The model under review builds one solid part; all positions refer to its coordinate system, in mm. Face numbers are marked on the shaded views. A direction names the side the tool comes from. Round coordinates to 2 decimals unless told otherwise and drop trailing zeros. Order: outer loops, then holes, each group sorted by start corner. A loop starts at its lowest first (then second) coordinate and runs counter-clockwise, first axis right, second up. Notation, with made-up numbers: (88, 3.5) -> (120, 3.5) arc R32 ccw to (120, 38.5) -> close; hole circle Ø1 at (-14.75, -12.5). An arc over 180 degrees is marked (long way). Return JSON: item names as keys, results as strings. Group by question number.
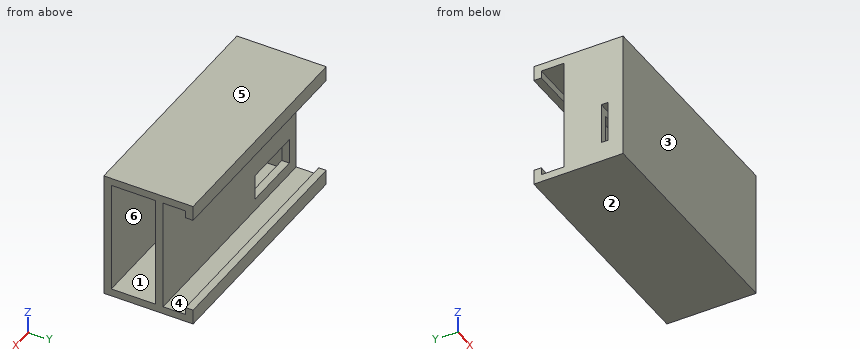
from build123d import *

# Parameters (mm, degrees)
SKETCH1_W            = 155
SKETCH1_H            = 85
BOSS_EXTRUDE1_DEPTH  = 5
SKETCH2_W            = 54
SKETCH2_H            = 35.4
BOSS_EXTRUDE19_DEPTH = 5
SKETCH14_W           = 5
SKETCH14_H           = 35.4
BOSS_EXTRUDE23_DEPTH = 9
SKETCH17_W           = 49
SKETCH17_H           = 4
BOSS_EXTRUDE24_DEPTH = 9
SKETCH18_W           = 49
SKETCH18_H           = 4.5
BOSS_EXTRUDE25_DEPTH = 5
SKETCH19_W           = 17.4
SKETCH19_H           = 4.5
BOSS_EXTRUDE26_DEPTH = 5
SKETCH20_W           = 49
SKETCH20_H           = 4
BOSS_EXTRUDE27_DEPTH = 9
SKETCH21_W           = 49
SKETCH21_H           = 4.5
BOSS_EXTRUDE28_DEPTH = 9
SKETCH24_W           = 40
SKETCH24_H           = 5.3
CUT_EXTRUDE3_DEPTH   = 9
SKETCH26_W           = 155
SKETCH26_H           = 5
BOSS_EXTRUDE29_DEPTH = 54.5
SKETCH27_W           = 155
SKETCH27_H           = 5
BOSS_EXTRUDE30_DEPTH = 75
SKETCH28_W           = 155
SKETCH28_H           = 5
BOSS_EXTRUDE31_DEPTH = 54.5
SKETCH29_W           = 75
SKETCH29_H           = 34.5
BOSS_EXTRUDE32_DEPTH = 5
SKETCH30_W           = 40
SKETCH30_H           = 17
CUT_EXTRUDE4_DEPTH   = 5
SKETCH31_W           = 27.4
SKETCH31_H           = 4.5
CUT_EXTRUDE6_DEPTH   = 5
SKETCH32_W           = 155
SKETCH32_H           = 5
BOSS_EXTRUDE33_DEPTH = 10
SKETCH33_W           = 155
SKETCH33_H           = 5
BOSS_EXTRUDE34_DEPTH = 10


with BuildPart() as part:
    # Sketch1 → Boss-Extrude1 (new body)
    with BuildSketch(Plane(origin=(0, 0, 0), x_dir=(1, 0, 0), z_dir=(0, 1, 0))):
        with Locations((48.537611559, -27.765767023)):
            Rectangle(SKETCH1_W, SKETCH1_H)
    extrude(amount=BOSS_EXTRUDE1_DEPTH)

    # Sketch2 → Boss-Extrude19 (add)
    with BuildSketch(Plane(origin=(0, 5, 0), x_dir=(1, 0, 0), z_dir=(0, 1, 0))):
        with Locations((3.037611559, -12.265767023)):
            Rectangle(SKETCH2_W, SKETCH2_H)
    extrude(amount=BOSS_EXTRUDE19_DEPTH)

    # Sketch14 → Boss-Extrude23 (add)
    with BuildSketch(Plane(origin=(0, 10, 0), x_dir=(1, 0, 0), z_dir=(0, 1, 0))):
        with Locations((27.537611559, -12.265767023)):
            Rectangle(SKETCH14_W, SKETCH14_H)
    extrude(amount=BOSS_EXTRUDE23_DEPTH)

    # Sketch17 → Boss-Extrude24 (add)
    with BuildSketch(Plane(origin=(0, 10, 0), x_dir=(1, 0, 0), z_dir=(0, 1, 0))):
        with Locations((0.537611559, 3.434232977)):
            Rectangle(SKETCH17_W, SKETCH17_H)
    extrude(amount=BOSS_EXTRUDE24_DEPTH)

    # Sketch18 → Boss-Extrude25 (add)
    with BuildSketch(Plane.XY.offset(-1.434232977)):
        with Locations((0.537611559, 16.75)):
            Rectangle(SKETCH18_W, SKETCH18_H)
    extrude(amount=BOSS_EXTRUDE25_DEPTH)

    # Sketch19 → Boss-Extrude26 (add)
    with BuildSketch(Plane.ZY.offset(-25.037611559)):
        with Locations((12.265767023, 16.75)):
            Rectangle(SKETCH19_W, SKETCH19_H)
    extrude(amount=BOSS_EXTRUDE26_DEPTH)

    # Sketch20 → Boss-Extrude27 (add)
    with BuildSketch(Plane(origin=(0, 10, 0), x_dir=(1, 0, 0), z_dir=(0, 1, 0))):
        with Locations((0.537611559, -27.965767023)):
            Rectangle(SKETCH20_W, SKETCH20_H)
    extrude(amount=BOSS_EXTRUDE27_DEPTH)

    # Sketch21 → Boss-Extrude28 (add)
    with BuildSketch(Plane.XY.offset(29.965767023)):
        with Locations((0.537611559, 16.75)):
            Rectangle(SKETCH21_W, SKETCH21_H)
    extrude(amount=-BOSS_EXTRUDE28_DEPTH)

    # Sketch24 → Cut-Extrude3 (cut)
    with BuildSketch(Plane(origin=(0, 19, 0), x_dir=(1, 0, 0), z_dir=(0, 1, 0))):
        with Locations((-0.962388441, -0.915767023)):
            Rectangle(SKETCH24_W, SKETCH24_H)
    extrude(amount=-CUT_EXTRUDE3_DEPTH, mode=Mode.SUBTRACT)

    # Sketch26 → Boss-Extrude29 (add)
    with BuildSketch(Plane(origin=(0, 5, 0), x_dir=(1, 0, 0), z_dir=(0, 1, 0))):
        with Locations((48.537611559, 12.234232977)):
            Rectangle(SKETCH26_W, SKETCH26_H)
    extrude(amount=BOSS_EXTRUDE29_DEPTH)

    # Sketch27 → Boss-Extrude30 (add)
    with BuildSketch(Plane.XY.offset(-9.734232977)):
        with Locations((48.537611559, 37)):
            Rectangle(SKETCH27_W, SKETCH27_H)
    extrude(amount=BOSS_EXTRUDE30_DEPTH)

    # Sketch28 → Boss-Extrude31 (add)
    with BuildSketch(Plane(origin=(0, 5, 0), x_dir=(1, 0, 0), z_dir=(0, 1, 0))):
        with Locations((48.537611559, -67.765767023)):
            Rectangle(SKETCH28_W, SKETCH28_H)
    extrude(amount=BOSS_EXTRUDE31_DEPTH)

    # Sketch29 → Boss-Extrude32 (add)
    with BuildSketch(Plane.ZY.offset(28.962388441)):
        with Locations((27.765767023, 22.25)):
            Rectangle(SKETCH29_W, SKETCH29_H)
    extrude(amount=-BOSS_EXTRUDE32_DEPTH)

    # Sketch30 → Cut-Extrude4 (cut)
    with BuildSketch(Plane(origin=(0, 39.5, 0), x_dir=(1, 0, 0), z_dir=(0, 1, 0))):
        with Locations((-0.962388441, -6.765767023)):
            Rectangle(SKETCH30_W, SKETCH30_H)
    extrude(amount=-CUT_EXTRUDE4_DEPTH, mode=Mode.SUBTRACT)

    # Sketch31 → Cut-Extrude6 (cut)
    with BuildSketch(Plane.ZY.offset(28.962388441)):
        with Locations((12.265767023, 12.25)):
            Rectangle(SKETCH31_W, SKETCH31_H)
    extrude(amount=-CUT_EXTRUDE6_DEPTH, mode=Mode.SUBTRACT)

    # Sketch32 → Boss-Extrude33 (add)
    with BuildSketch(Plane.XY.offset(70.265767023)):
        with Locations((48.537611559, 57)):
            Rectangle(SKETCH32_W, SKETCH32_H)
    extrude(amount=-BOSS_EXTRUDE33_DEPTH)

    # Sketch33 → Boss-Extrude34 (add)
    with BuildSketch(Plane(origin=(0, 0, -14.734232977), x_dir=(-1, 0, 0), z_dir=(0, 0, -1))):
        with Locations((-48.537611559, 57)):
            Rectangle(SKETCH33_W, SKETCH33_H)
    extrude(amount=-BOSS_EXTRUDE34_DEPTH)


solid = part.part
Item 1: Consider section C-C on y = 30. State the section outline as (x, z) points.
Item 2: Consider section D-D on y = 7. State the section outline as (x, z) points.
Item 3: Wall thickness on line 1 along Z through (x, y) = (117, 44.5); line 2 along Y through (x, z) = (68.5, 64.5); line 3 along Y through (x, z) = (53.5, 39): over which ranges is each line inside the solid? List them lowest first.
Item 4: For the marked faces 4, 5 and 6, list the 3-axis set-ups (+Z, -Z, +X, -X, +Y, -Y) from which the entire face can be reached by the end or side of a thin tool; tool diameter is ignored.
Item 5: Insertion check: pin 1 Ø5 at (y, z) = (31, 13) entering from +X; pin 2 Ø5 at (x, z) = (-13, 18) entering from +Y; pin 3 Ø2 at (x, z) = (23.5, 38.5) entering from -Y. Each pin has a flat end and moves straight along its axis. Give the tip position at first contact, or say it passes through.
Item 6: Consider section A-A on x = 58. State the section outline as (y, z) points.
Item 7: The part is to be moulded in two halves that separate along Z. For the marked faces 1, 2 and 3, say which applies: +Z half, -Z half, draft (parallel to the pull), parting line (faces both ways), or undercut.
Values:
{
 "1": {"outline": "(-28.96, -14.73) -> (126.04, -14.73) -> (126.04, -9.73) -> (-23.96, -9.73) -> (-23.96, 65.27) -> (126.04, 65.27) -> (126.04, 70.27) -> (-28.96, 70.27) -> close"},
 "2": {"outline": "(-28.96, -14.73) -> (126.04, -14.73) -> (126.04, -9.73) -> (-23.96, -9.73) -> (-23.96, -5.43) -> (30.04, -5.43) -> (30.04, 29.97) -> (-23.96, 29.97) -> (-23.96, 65.27) -> (126.04, 65.27) -> (126.04, 70.27) -> (-28.96, 70.27) -> close"},
 "3": {"line 1": "-14.73 to -9.73, 65.27 to 70.27", "line 2": "0 to 5, 34.5 to 39.5, 54.5 to 59.5", "line 3": "0 to 5, 34.5 to 39.5"},
 "4": {"face 4": "+X, -X", "face 5": "+Z, +X, -X, +Y, -Y", "face 6": "+X"},
 "5": {"pin 1": "x = -23.96", "pin 2": "y = 39.5", "pin 3": "y = 0"},
 "6": {"outline": "(0, -14.73) -> (59.5, -14.73) -> (59.5, -4.73) -> (54.5, -4.73) -> (54.5, -9.73) -> (39.5, -9.73) -> (39.5, 65.27) -> (54.5, 65.27) -> (54.5, 60.27) -> (59.5, 60.27) -> (59.5, 70.27) -> (0, 70.27) -> close; hole (5, -9.73) -> (34.5, -9.73) -> (34.5, 65.27) -> (5, 65.27) -> close"},
 "7": {"face 1": "undercut", "face 2": "-Z half", "face 3": "draft"}
}
